```python
from build123d import *

# Parameters (mm, degrees)
SKETCH1_W           = 112
SKETCH1_H           = 58
BOSS_EXTRUDE1_DEPTH = 0.8
SKETCH2_W           = 112
SKETCH2_H           = 58
SKETCH2_W_2         = 110
SKETCH2_H_2         = 56
BOSS_EXTRUDE2_DEPTH = 28
SKETCH3_R           = 1.75
CUT_EXTRUDE1_DEPTH  = 28
BOSS_EXTRUDE3_START = 2
SKETCH4_R           = 3.25
SKETCH4_R_2         = 1.75
BOSS_EXTRUDE3_DEPTH = 2
CUT_EXTRUDE2_DEPTH  = 2
CUT_EXTRUDE3_DEPTH  = 72
BOSS_EXTRUDE4_DEPTH = 28.8
SKETCH8_W           = 11.5
SKETCH8_H           = 1.5
CUT_EXTRUDE4_DEPTH  = 70


with BuildPart() as part:
    # Sketch1 → Boss-Extrude1 (new body)
    with BuildSketch(Plane(origin=(0, 0, 0), x_dir=(1, 0, 0), z_dir=(0, 1, 0))):
        Rectangle(SKETCH1_W, SKETCH1_H)
    extrude(amount=BOSS_EXTRUDE1_DEPTH)

    # Sketch2 → Boss-Extrude2 (add)
    with BuildSketch(Plane(origin=(0, 0.8, 0), x_dir=(1, 0, 0), z_dir=(0, 1, 0))):
        Rectangle(SKETCH2_W, SKETCH2_H)
        Rectangle(SKETCH2_W_2, SKETCH2_H_2, mode=Mode.SUBTRACT)
    extrude(amount=BOSS_EXTRUDE2_DEPTH)

    # Sketch3 → Cut-Extrude1 (cut)
    with BuildSketch(Plane(origin=(0, 0.8, 0), x_dir=(1, 0, 0), z_dir=(0, 1, 0))):
        with Locations(Location((-36, 25.5, 0), (0, 0, 270))):
            Circle(SKETCH3_R)
        with Locations(Location((-36, -25.5, 0), (0, 0, 270))):
            Circle(SKETCH3_R)
        with Locations(Location((45.5, 25.5, 0), (0, 0, 270))):
            Circle(SKETCH3_R)
        with Locations(Location((45.5, -25.5, 0), (0, 0, 270))):
            Circle(SKETCH3_R)
    extrude(amount=-CUT_EXTRUDE1_DEPTH, mode=Mode.SUBTRACT)

    # Sketch4 → Boss-Extrude3 (add)
    # profile 1 of 4: a face of its own
    with BuildSketch(Plane(origin=(0, 0.8, 0), x_dir=(1, 0, 0), z_dir=(0, 1, 0)).offset(BOSS_EXTRUDE3_START)):
        with Locations((-36, 25.5)):
            Circle(SKETCH4_R)
        with Locations(Location((-36, 25.5, 0), (0, 0, 270))):
            Circle(SKETCH4_R_2, mode=Mode.SUBTRACT)
    # profile 2 of 4: a face of its own
    with BuildSketch(Plane(origin=(0, 0.8, 0), x_dir=(1, 0, 0), z_dir=(0, 1, 0)).offset(BOSS_EXTRUDE3_START)):
        with Locations((45.5, 25.5)):
            Circle(SKETCH4_R)
        with Locations(Location((45.5, 25.5, 0), (0, 0, 270))):
            Circle(SKETCH4_R_2, mode=Mode.SUBTRACT)
    # profile 3 of 4: a face of its own
    with BuildSketch(Plane(origin=(0, 0.8, 0), x_dir=(1, 0, 0), z_dir=(0, 1, 0)).offset(BOSS_EXTRUDE3_START)):
        with Locations((-36, -25.5)):
            Circle(SKETCH4_R)
        with Locations(Location((-36, -25.5, 0), (0, 0, 270))):
            Circle(SKETCH4_R_2, mode=Mode.SUBTRACT)
    # profile 4 of 4: a face of its own
    with BuildSketch(Plane(origin=(0, 0.8, 0), x_dir=(1, 0, 0), z_dir=(0, 1, 0)).offset(BOSS_EXTRUDE3_START)):
        with Locations((45.5, -25.5)):
            Circle(SKETCH4_R)
        with Locations(Location((45.5, -25.5, 0), (0, 0, 270))):
            Circle(SKETCH4_R_2, mode=Mode.SUBTRACT)
    extrude(amount=-BOSS_EXTRUDE3_DEPTH)

    # Sketch5 → Cut-Extrude2 (cut)
    with BuildSketch(Plane(origin=(-55, 0, 0), x_dir=(0, 0, -1), z_dir=(1, 0, 0))):
        with BuildLine():
            Line((-10.5, 28.8), (-10.5, 10.8))
            ThreePointArc((-10.5, 10.8), (-8, 8.3), (-5.5, 10.8))
            Line((-5.5, 10.8), (-5.5, 28.8))
            Line((-5.5, 28.8), (-10.5, 28.8))
        make_face()
    extrude(amount=-CUT_EXTRUDE2_DEPTH, mode=Mode.SUBTRACT)

    # Sketch6 → Cut-Extrude3 (cut)
    with BuildSketch(Plane.XY.offset(29)):
        with BuildLine():
            Line((34.5, 25.8), (34.5, 28.8))
            Line((34.5, 28.8), (37.5, 28.8))
            Line((37.5, 28.8), (37.5, 25.8))
            ThreePointArc((37.5, 25.8), (36, 24.3), (34.5, 25.8))
        make_face()
    extrude(amount=-CUT_EXTRUDE3_DEPTH, mode=Mode.SUBTRACT)

    # Sketch7 → Boss-Extrude4 (add)
    with BuildSketch(Plane.XZ):
        Polygon((-41, 29), (-38, 32), (-34, 32), (-31, 29), align=None)
        Polygon((40.5, 29), (43.5, 32), (47.5, 32), (50.5, 29), align=None)
        Polygon((-41, -29), (-38, -32), (-34, -32), (-31, -29), align=None)
        Polygon((40.5, -29), (43.5, -32), (47.5, -32), (50.5, -29), align=None)
    extrude(amount=-BOSS_EXTRUDE4_DEPTH)

    # Sketch8 → Cut-Extrude4 (cut)
    with BuildSketch(Plane.XY.offset(29)):
        with Locations((4.75, 26.55)):
            Rectangle(SKETCH8_W, SKETCH8_H)
    extrude(amount=-CUT_EXTRUDE4_DEPTH, mode=Mode.SUBTRACT)


solid = part.part
```
Part model, mm, in its own coordinate system. A direction names the side the tool comes from. Round coordinates to 2 decimals unless told otherwise and drop trailing zeros. Write each loop counter-clockwise with the first axis right and the second up, starting at its lowest first coordinate (ties: lowest second). Pieces come first, ordered by that corner, then holes.
Item 1: Which spindle directions (+Z, -Z, +X, -X, +Y, -Y) get a long thin tool onto all of the face, cutting with end or side? Do faces 1 (the flat face through (42, 14.2, 30.5)), 2 (the flat face through (53, 14, 29)), 3 (the flat face through (-37.5, 2.8, -23.9)), 4 (the flat face through (-49, 14, -29)). Say none if no direction does.
Results:
face 1: +Z, +Y, -Y
face 2: +Z, +X, +Y, -Y
face 3: +Y
face 4: -Z, -X, +Y, -Y
Item 2: Cut at A-A, the plane x = 7.5. Give the cut face in (y, z).
Results:
outline: (0, -29) - (25.8, -29) - (25.8, -28) - (0.8, -28) - (0.8, 28) - (25.8, 28) - (25.8, 29) - (0, 29) - close; (27.3, -29) - (28.8, -29) - (28.8, -28) - (27.3, -28) - close; (27.3, 28) - (28.8, 28) - (28.8, 29) - (27.3, 29) - close
Item 3: Cut at C-C, the plane y = 15.25. Give the cut face in (x, z).
Results:
outline: (-56, -29) - (-41, -29) - (-38, -32) - (-34, -32) - (-31, -29) - (40.5, -29) - (43.5, -32) - (47.5, -32) - (50.5, -29) - (56, -29) - (56, 29) - (50.5, 29) - (47.5, 32) - (43.5, 32) - (40.5, 29) - (-31, 29) - (-34, 32) - (-38, 32) - (-41, 29) - (-56, 29) - (-56, 10.5) - (-55, 10.5) - (-55, 28) - (55, 28) - (55, -28) - (-55, -28) - (-55, 5.5) - (-56, 5.5) - close
Item 4: Drop flat-ended pins along their axis: pin 1 Ø4 at (x, z) = (-36, 25.5) entering from +Y; pin 2 Ø17 at (x, z) = (18.5, -0.5) entering from +Y; pin 3 Ø3 at (x, y) = (17.5, 6.5) entering from -Z. Give the stop position or say it passes through.
Results:
pin 1: stops at y = 2.8
pin 2: stops at y = 0.8
pin 3: stops at z = -29
Item 5: Cut at D-D, the plane x = -19. Give the cut face in (y, z), plus the area to 3 significant figures.
Results:
outline: (0, -29) - (28.8, -29) - (28.8, -28) - (0.8, -28) - (0.8, 28) - (28.8, 28) - (28.8, 29) - (0, 29) - close
area: 102 mm2
Item 6: Probe L1, parallel to X at y = 0.65, z = 25.5; L2, parallel to X at y = 1.3, z = 25.5; L3, parallel to X at y = 19.25, z = 27.5. List the from-to ranges inside material, lowest first.
Results:
L1: x = -56 to -37.75, -34.25 to 43.75, 47.25 to 56
L2: x = -56 to -55, -39.25 to -37.75, -34.25 to -32.75, 42.25 to 43.75, 47.25 to 48.75, 55 to 56
L3: x = -56 to -55, 55 to 56
Item 7: Two-plate mould, pull along X, no slides. Class faces 5 (the flat face through (49, 14.2, 30.5)), 6 (the flat face through (-40, 14, -30)), 7 (the flat face through (-1, 0, 0)), 8 (the flat face through (55, 15, 0)): +X half, -X half, draft (parallel to the pull), parting line (faces both ways), or undercut.
Results:
face 5: +X half
face 6: -X half
face 7: draft
face 8: undercut
Item 8: Cut at B-B, the plane z = -8. Give the cut face in (x, y).
Results:
outline: (-56, 0) - (56, 0) - (56, 28.8) - (55, 28.8) - (55, 0.8) - (-55, 0.8) - (-55, 28.8) - (-56, 28.8) - close
